Autodesk Inventor part; units mm, degrees
ref_plane "YZ Plane" through (0, 0, 0) normal (1, 0, 0) x (0, 1, 0)
ref_plane "XZ Plane" through (0, 0, 0) normal (0, 1, 0) x (-1, 0, 0)
ref_plane "XY Plane" through (0, 0, 0) normal (0, 0, 1) x (1, 0, 0)
sketch "Sketch1" plane through (0, 0, 0) normal (1, 0, 0) x (0, 1, 0)
  line L0 (1.8986, 1.3831) -> (-40.1014, 1.3831)
  line L1 (-40.1014, 1.3831) -> (-40.1014, -42.3731)
  line L2 (-40.1014, -42.3731) -> (1.8986, -42.3731)
  line L3 (1.8986, -42.3731) -> (1.8986, 1.3831)
  point P0 (0, 0)
  dimension "d0" = 42
extrude "Extrusion1" add sketch "Sketch1" along normal blind 100
sketch "Sketch3" plane through (0, 0, 0) normal (-1, 0, 0) x (0, 0, 1)
  point P0 (0, 0)
sketch "Sketch8" plane through (0, 0, 0) normal (-1, 0, 0) x (0, 0, 1)
  point P0 (0, 0)
  point P1 (-20.6894, -17.7504)
hole "Hole4" at (0, -17.7504, -20.6894) direction (1, 0, 0) diameter 15.875 end through all
sketch "Sketch9" plane through (0, -40.1014, 1.3831) normal (0, 0, 1) x (1, 0, 0)
  line L0 (0, 42) -> (100, 42)
  line L1 (0, 0) -> (100, 0)
  line L2 (1.351, 42) -> (99.1356, 42)
  line L3 (99.1356, 42) -> (99.1356, 0)
  line L4 (99.1356, 0) -> (1.351, 0)
  line L5 (1.351, 0) -> (1.351, 42)
  point P0 (0, 40.1014)
  point P1 (1.351, 0)
extrude "Extrusion4" cut sketch "Sketch9" against normal blind 42
properties part number "clamp 2"
Check sheet for the modelled part. Datum: model origin and axes. Units: mm. A direction names the side the tool comes from. Coordinates: 2 decimals unless noted, no trailing zeros. Order: outer loops, then holes, each group sorted by start corner. A loop starts at its lowest first (then second) coordinate and runs counter-clockwise, first axis right, second up. Notation, with made-up numbers: (-37, 44) -> (19, 44) arc R26 ccw to (19, 72) -> close; hole circle Ø10 at (-14, 64). An arc over 180 degrees is marked (long way). Write each question's results on one line, items separated by ' | '. Start each with the question number.
1) Depth check by flat-ended pin: pin 1 (12 mm diameter, centred on x = 29.5, y = -23.5, fed in from +Z). Enter the tip coordinate at first touch or a pass-through.
2) Section check B-B (y = -11). Enter the section's corners in (x, z), and give its area (3 significant figures).
3) Section check A-A (z = -5.5). Enter the section's corners in (x, y), and give its area (3 significant figures).
4) Set-up check for faces 4 (the face through (50, -19, -40.617)), 5 (the face through (50, -40.101, -41)): record each of +Z, -Z, +X, -X, +Y, -Y from which the full face is reachable in a straight line by a thin tool's end or side.
5) Section check D-D (y = -6.5). Enter the section's corners in (x, z).
6) Material ranges on line 1 along X through (y, z) = (-20, -3.5); line 2 along Z through (x, y) = (79, -31.5), recorded low to high.
7) Section check C-C (z = -15). Enter the section's corners in (x, y), and give its area (3 significant figures).
8) Draft check along X on faces 1 (the face through (0, -24, -15)), 2 (the face through (99.57, -18.1, -28.62)), 3 (the face through (1.351, -24, -15)). Enter one of: pulls with the +X half, pulls with the -X half, needs draft (parallel to the pull), parting line crosses it, or undercut.
Checked values:
1) pin 1: z = -40.62
2) outline: (0, -42.37) -> (100, -42.37) -> (100, -24.87) -> (99.14, -24.87) -> (99.14, -40.62) -> (1.35, -40.62) -> (1.35, -24.87) -> (0, -24.87) -> close; (0, -16.51) -> (1.35, -16.51) -> (1.35, 1.38) -> (0, 1.38) -> close; (99.14, -16.51) -> (100, -16.51) -> (100, 1.38) -> (99.14, 1.38) -> close | area: 250 mm²
3) outline: (0, -40.1) -> (1.35, -40.1) -> (1.35, 1.9) -> (0, 1.9) -> close; (99.14, -40.1) -> (100, -40.1) -> (100, 1.9) -> (99.14, 1.9) -> close | area: 93.0 mm²
4) face 4: +Z, +Y, -Y | face 5: +Z, -Z, +X, -X, -Y
5) outline: (0, -42.37) -> (100, -42.37) -> (100, 1.38) -> (99.14, 1.38) -> (99.14, -40.62) -> (1.35, -40.62) -> (1.35, 1.38) -> (0, 1.38) -> close
6) line 1: 0 to 1.35, 99.14 to 100 | line 2: -42.37 to -40.62
7) outline: (0, -40.1) -> (1.35, -40.1) -> (1.35, -23.29) -> (0, -23.29) -> close; (0, -12.22) -> (1.35, -12.22) -> (1.35, 1.9) -> (0, 1.9) -> close; (99.14, -40.1) -> (100, -40.1) -> (100, -23.29) -> (99.14, -23.29) -> close; (99.14, -12.22) -> (100, -12.22) -> (100, 1.9) -> (99.14, 1.9) -> close | area: 68.5 mm²
8) face 1: pulls with the -X half | face 2: needs draft | face 3: undercut
